from build123d import *

# Parameters (mm, degrees)
SKETCH_1_W          = 100
SKETCH_1_H          = 60
EXTRUDE_1_DEPTH     = 3.2
SKETCH_2_R          = 12.5
SKETCH_2_R_2        = 1.6
SKETCH_2_R_3        = 1.5
SKETCH_2_R_4        = 5.75
CUT_EXTRUDE_1_DEPTH = 3.2
FILLET_1_R          = 2
FILLET_2_R          = 1


with BuildPart() as part:
    # 草图1 → 凸台-拉伸1 (new body)
    with BuildSketch(Plane(origin=(0, 0, 0), x_dir=(1, 0, 0), z_dir=(0, 1, 0))):
        Polygon((-57.5, -15), (-60.328427125, -15), (-65, -15), (-65, -30), (-50, -30), (-50, -15), align=None)
        Rectangle(SKETCH_1_W, SKETCH_1_H)
        Polygon((-50, -7.5), (-50, -4.671572875), (-60.328427125, -15), (-57.5, -15), align=None)
        Polygon((65, -15), (60.328427125, -15), (57.5, -15), (50, -15), (50, -30), (65, -30), align=None)
        Polygon((60.328427125, -15), (50, -4.671572875), (50, -7.5), (57.5, -15), align=None)
    extrude(amount=EXTRUDE_1_DEPTH)

    # 草图2 → 切除-拉伸1 (cut)
    with BuildSketch(Plane(origin=(0, 3.2, 0), x_dir=(1, 0, 0), z_dir=(0, 1, 0))):
        with Locations(Location((0, -6.443650814, 0), (0, 0, 270))):
            Circle(SKETCH_2_R)
        with Locations(Location((15.556349186, -22, 0), (0, 0, 270))):
            Circle(SKETCH_2_R_2)
        with Locations(Location((15.556349186, 9.112698372, 0), (0, 0, 270))):
            Circle(SKETCH_2_R_2)
        with Locations(Location((-15.556349186, 9.112698372, 0), (0, 0, 270))):
            Circle(SKETCH_2_R_2)
        with Locations(Location((-15.556349186, -22, 0), (0, 0, 270))):
            Circle(SKETCH_2_R_2)
        with Locations(Location((-47.5, 20, 0), (0, 0, 270))):
            Circle(SKETCH_2_R_3)
        with Locations(Location((-47.5, -20, 0), (0, 0, 270))):
            Circle(SKETCH_2_R_3)
        with Locations(Location((47.5, -20, 0), (0, 0, 270))):
            Circle(SKETCH_2_R_3)
        with Locations(Location((47.5, 20, 0), (0, 0, 270))):
            Circle(SKETCH_2_R_3)
        with Locations(Location((-57.5, -22.5, 0), (0, 0, 270))):
            Circle(SKETCH_2_R_4)
        with Locations(Location((57.5, -22.5, 0), (0, 0, 270))):
            Circle(SKETCH_2_R_4)
        with Locations(Location((30, 19, 0), (0, 0, 270))):
            Circle(SKETCH_2_R_3)
        with Locations(Location((30, 11, 0), (0, 0, 270))):
            Circle(SKETCH_2_R_3)
        with Locations(Location((-30, 11, 0), (0, 0, 270))):
            Circle(SKETCH_2_R_3)
        with Locations(Location((-30, 19, 0), (0, 0, 270))):
            Circle(SKETCH_2_R_3)
        with Locations(Location((30, -11, 0), (0, 0, 270))):
            Circle(SKETCH_2_R_3)
        with Locations(Location((30, -19, 0), (0, 0, 270))):
            Circle(SKETCH_2_R_3)
        with Locations(Location((-30, -19, 0), (0, 0, 270))):
            Circle(SKETCH_2_R_3)
        with Locations(Location((-30, -11, 0), (0, 0, 270))):
            Circle(SKETCH_2_R_3)
    extrude(amount=-CUT_EXTRUDE_1_DEPTH, mode=Mode.SUBTRACT)

    # 圆角1
    fillet_1_edges = [part.edges().sort_by_distance(p)[0] for p in [
        (-60.328427125, 1.6, 15),
        (-50, 1.6, 4.671572875),
        (-50, 1.6, -30),
        (50, 1.6, -30),
        (50, 1.6, 4.671572875),
        (60.328427125, 1.6, 15),
        (65, 1.6, 15),
        (65, 1.6, 30),
        (-65, 1.6, 30),
        (-65, 1.6, 15),
    ]]
    fillet(fillet_1_edges, radius=FILLET_1_R)

    # 圆角2
    fillet_2_edges = [part.edges().sort_by_distance(p)[0] for p in [
        (-57.5, 1.6, 15),
        (-50, 1.6, 15),
        (-50, 1.6, 7.5),
        (50, 1.6, 7.5),
        (50, 1.6, 15),
        (57.5, 1.6, 15),
    ]]
    fillet(fillet_2_edges, radius=FILLET_2_R)


solid = part.part
Input: part model. Units: mm. Frame: model coordinates. A direction names the side the tool comes from. Give positions to 0.01 mm unless a question says otherwise; leave off trailing zeros. Order: outer loops, then holes, each group sorted by start corner. A loop starts at its lowest first (then second) coordinate and runs counter-clockwise, first axis right, second up. Notation, with made-up numbers: M 81.25,66 L 95.25,66 A23 cw 95.25,92 Z; hole C 78,50 d1. An arc over 180 degrees is marked long. Answer as a JSON object with one key per item and string values.
1. Cut plane C-C, the plane y = 0.7. State how many separate pieces and enclosed holes the cut face has, and give its area (3 significant figures).
Result sheet:
{"separate pieces": "1", "enclosed holes": "21", "area": "5,690 mm²"}
2. Reachability of faces 4 (the flat face through (-1, 2, -30)), 5 (the flat face through (50, 2, -12)), 6 (the flat face through (50, 2, 12)) from +Z, -Z, +X, -X, +Y, -Y: full face, straight path, thin tool, end or side. Return the list, or none.
Result sheet:
{"face 4": "-Z, +X, -X, +Y, -Y", "face 5": "-Z, +X, +Y, -Y", "face 6": "+Y, -Y"}
3. Pull-direction query (X, two-part tool) for faces 1 (the cylindrical face through (61.386, 1.622, 18.262)), 2 (the flat face through (65, 2, 23)), 3 (the flat face through (-65, 2, 22)); classes: +X half, -X half, draft (parallel to the pull), parting line (faces both ways), or undercut.
Result sheet:
{"face 1": "undercut", "face 2": "+X half", "face 3": "-X half"}
4. Cut plane A-A, the plane x = -30. Output: boundary loops of the cut face in (y, z).
Result sheet:
{"outline": "M 0,-30 L 3.2,-30 L 3.2,-20.5 L 0,-20.5 Z; M 0,-17.5 L 3.2,-17.5 L 3.2,-12.5 L 0,-12.5 Z; M 0,-9.5 L 3.2,-9.5 L 3.2,9.5 L 0,9.5 Z; M 0,12.5 L 3.2,12.5 L 3.2,17.5 L 0,17.5 Z; M 0,20.5 L 3.2,20.5 L 3.2,30 L 0,30 Z"}
5. Ray query, line 1 (Z direction, x = -16.5, y = 2.2); line 2 (X direction, y = 1.2, z = -20); line 3 (X direction, y = 2.2, z = 13). Return the intervals inside material, ascending. Write a range as [from, to].
Result sheet:
{"line 1": "[-30, -10.4], [-7.82, 20.71], [23.29, 30]", "line 2": "[-50, -49], [-46, -31.12], [-28.88, 28.88], [31.12, 46], [49, 50]", "line 3": "[-58.33, -55.5], [-50, -10.64], [10.64, 50], [55.5, 58.33]"}
6. First-contact query: P1, Ø1, axis at y = 2, z = -20, coming from the +X side; P2, Ø1, axis at y = 1, z = 11, coming from the -X side; P3, Ø3.5, axis at x = 47.5, z = 20, coming from the +Y side; P4, Ø1.6, axis at x = -53, y = 1.5, coming from the -Z side. Flat tips, straight axial feed; report the tip coordinate or a pass-through.
Result sheet:
{"P1": "x = 50", "P2": "x = -56.83", "P3": "y = 3.2", "P4": "z = 6.87"}
7. Cut plane B-B, the plane x = -57.5. Output: boundary loops of the cut face in (y, z).
Result sheet:
{"outline": "M 0,12.17 L 3.2,12.17 L 3.2,16.75 L 0,16.75 Z; M 0,28.25 L 3.2,28.25 L 3.2,30 L 0,30 Z"}
